Geometry: final body of the model. Coordinates: model frame, mm. A direction names the side the tool comes from. Give positions to 0.01 mm unless a question says otherwise; leave off trailing zeros. Order: outer loops, then holes, each group sorted by start corner. A loop starts at its lowest first (then second) coordinate and runs counter-clockwise, first axis right, second up. Notation, with made-up numbers: M -37.75,48 L -18.75,48 A30 cw -18.75,74 Z; hole C -32,-32.75 d2. An arc over 180 degrees is marked long. Use CSV: the item, a comma, the result in double quotes.
```python
from build123d import *

# Parameters (mm, degrees)
SKETCH_1_W          = 42.72
SKETCH_1_H          = 60.26
EXTRUDE_1_DEPTH     = 2.2
SKETCH_2_W          = 36.72
SKETCH_2_H          = 48.96
CUT_EXTRUDE_1_DEPTH = 0.1
SKETCH_3_W          = 29.464595321
SKETCH_3_H          = 0.5
EXTRUDE_1004_DEPTH  = 29
SKETCH_4_W          = 16.518374104
SKETCH_4_H          = 17.022875601
SKETCH_4_W_2        = 6.622613049
SKETCH_4_H_2        = 1.675281879
CUT_EXTRUDE_2_DEPTH = 44.9
FILLET_1_R          = 2


with BuildPart() as part:
    # Sketch 1 → Extrude 1 (new body)
    with BuildSketch(Plane.XY):
        Rectangle(SKETCH_1_W, SKETCH_1_H)
    extrude(amount=EXTRUDE_1_DEPTH)

    # Sketch 2 → Cut-Extrude 1 (cut)
    with BuildSketch(Plane.XY.offset(2.2)):
        with Locations((0, 2.74)):
            Rectangle(SKETCH_2_W, SKETCH_2_H)
    extrude(amount=-CUT_EXTRUDE_1_DEPTH, mode=Mode.SUBTRACT)

    # Sketch 3 → Extrude 1004 (add)
    with BuildSketch(Plane.XZ.offset(30.13)):
        with Locations((3.732297661, 0.45)):
            Rectangle(SKETCH_3_W, SKETCH_3_H)
    extrude(amount=EXTRUDE_1004_DEPTH)

    # Sketch 4 → Cut-Extrude 2 (cut)
    with BuildSketch(Plane.XY.offset(0.7)):
        with Locations((10.205408269, -50.6185622)):
            Rectangle(SKETCH_4_W, SKETCH_4_H)
        with Locations((11.972121528, -30.96764094)):
            Rectangle(SKETCH_4_W_2, SKETCH_4_H_2)
    extrude(amount=-CUT_EXTRUDE_2_DEPTH, mode=Mode.SUBTRACT)

    # Fillet 1
    fillet_1_edges = [part.edges().sort_by_distance(p)[0] for p in [
        (1.946221217, -42.107124399, 0.45),
        (18.464595321, -42.107124399, 0.45),
    ]]
    fillet(fillet_1_edges, radius=FILLET_1_R)


solid = part.part
```
1. Reachability of faces 1 (the face through (0, -41, 0.2)), 2 (the face through (0, 0, 0)), 3 (the face through (0, -41, 0.7)) from +Z, -Z, +X, -X, +Y, -Y: full face, straight path, thin tool, end or side. Return the list, or none.
Answer:
face 1,"-Z, +X, -X, -Y"
face 2,"-Z, +X, -X, +Y, -Y"
face 3,"+Z, +X, -X, -Y"
2. Pull-direction query (X, two-part tool) for faces 4 (the face through (0, 3, 2.1)), 5 (the face through (-21.36, 0, 1)), 6 (the face through (0, 30.13, 1)); classes: +X half, -X half, draft (parallel to the pull), parting line (faces both ways), or undercut.
Answer:
face 4,"undercut"
face 5,"-X half"
face 6,"draft"
3. Pin query (flat end, axial travel): pin 1 Ø12 at (x, y) = (-0.5, 8) entering from -Z; pin 2 Ø1.1 at (x, z) = (-7.5, 1.5) entering from -Y; pin 3 Ø0.5 at (y, z) = (-54, 0.5) entering from +X; pin 4 Ø1 at (x, y) = (-11, 10) entering from +Z. Return the tip coordinate at first contact, or that it passes through.
Answer:
pin 1,"z = 0"
pin 2,"y = -30.13"
pin 3,"x = 1.95"
pin 4,"z = 2.1"
4. Section D-D, the plane x = -17.5. Return the cut outline in (y, z), plus the area to 3 significant figures.
Answer:
outline,"M -30.13,0 L 30.13,0 L 30.13,2.2 L 27.22,2.2 L 27.22,2.1 L -21.74,2.1 L -21.74,2.2 L -30.13,2.2 Z"
area,"128 mm2"
5. Section B-B, the plane x = -5. Return the cut outline in (y, z).
Answer:
outline,"M -59.13,0.2 L -30.13,0.2 L -30.13,0 L 30.13,0 L 30.13,2.2 L 27.22,2.2 L 27.22,2.1 L -21.74,2.1 L -21.74,2.2 L -30.13,2.2 L -30.13,0.7 L -59.13,0.7 Z"
6. Line query: line 1 (Y direction, x = 15, z = 0.65); line 2 (Y direction, x = -14, z = 1.7); line 3 (Z direction, x = 12, y = 18.5). Output: solid intervals per line, ascending.
Answer:
line 1,"-42.11 to -31.81, -30.13 to 30.13"
line 2,"-30.13 to 30.13"
line 3,"0 to 2.1"
7. Section C-C, the plane z = 1.7. Return the cut outline in (x, y).
Answer:
outline,"M -21.36,-30.13 L 21.36,-30.13 L 21.36,30.13 L -21.36,30.13 Z"
8. Section A-A, the plane y = 21. Return the cut outline in (x, z), plus the area to 3 significant figures.
Answer:
outline,"M -21.36,0 L 21.36,0 L 21.36,2.2 L 18.36,2.2 L 18.36,2.1 L -18.36,2.1 L -18.36,2.2 L -21.36,2.2 Z"
area,"90.3 mm2"
